Can you work these out from the model? Positions are in its coordinate system, mm. A direction names the side the tool comes from. Coordinates: 2 decimals unless noted, no trailing zeros. Order: outer loops, then holes, each group sorted by start corner. A loop starts at its lowest first (then second) coordinate and runs counter-clockwise, first axis right, second up. Notation, with made-up numbers: (32.5, 68) -> (51.5, 68) arc R6 cw to (51.5, 72) -> close; hole circle Ø11 at (-8, 37.5). An arc over 180 degrees is marked (long way). Write item = value, one per line. Start each with the question number.
Autodesk Inventor part; units mm, degrees
ref_plane "YZ Plane" through (0, 0, 0) normal (1, 0, 0) x (0, 1, 0)
ref_plane "XZ Plane" through (0, 0, 0) normal (0, 1, 0) x (-1, 0, 0)
ref_plane "XY Plane" through (0, 0, 0) normal (0, 0, 1) x (1, 0, 0)
sketch "Sketch1" plane through (0, 0, 0) normal (0, 1, 0) x (-1, 0, 0)
  line L0 (2, 0) -> (23, 0)
  line L1 (25, -2) -> (25, -21.862)
  line L2 (23, -23.862) -> (2, -23.862)
  line L3 (0, -21.862) -> (0, -2)
  arc A0 (25, -2) -> (23, 0) centre (23, -2) ccw
  arc A1 (23, -23.862) -> (25, -21.862) centre (23, -21.862) ccw
  arc A2 (0, -21.862) -> (2, -23.862) centre (2, -21.862) ccw
  arc A3 (2, 0) -> (0, -2) centre (2, -2) ccw
  line L4 (23, 0) -> (23, -23.862) construction
  line L5 (2, -23.862) -> (2, 0) construction
  line L6 (25, -2) -> (0, -2) construction
  line L7 (0, -14.5) -> (25, -14.5) construction
  circle A4 centre (23, -2) radius 1.1
  circle A5 centre (23, -14.5) radius 1.1
  circle A6 centre (2, -14.5) radius 1.1
  circle A7 centre (2, -2) radius 1.1
  point P0 (0, 0)
  point P1 (25, -23.862)
  point P2 (25, 0)
  point P3 (0, -23.862)
  dimension "d0" = 25
  dimension "d1" = 23.862
  dimension "d2" = 2
  dimension "d3" = 2
  dimension "d4" = 14.5
  dimension "d5" = 2
  dimension "d6" = 2
  dimension "d7" = 2.2
  dimension "d8" = 2.2
  dimension "d9" = 2.2
  dimension "d10" = 2.2
extrude "Extrusion1" add sketch "Sketch1" along normal blind 1.2
sketch "Sketch2" plane through (0, 1.2, 0) normal (0, 1, 0) x (1, 0, 0)
  line L0 (-25, 21.862) -> (-25, 2) construction
  line L1 (-25, 11.931) -> (0, 11.931) construction
  line L2 (0, 2) -> (0, 21.862) construction
  line L3 (-2, 23.862) -> (-23, 23.862) construction
  line L4 (-12.5, 23.862) -> (-12.5, 0) construction
  line L5 (-23, 0) -> (-2, 0) construction
  line L6 (-16.75, 18.65) -> (-8.25, 18.65)
  line L7 (-8.25, 18.65) -> (-8.25, 10.15)
  line L8 (-8.25, 10.15) -> (-16.75, 10.15)
  line L9 (-16.75, 10.15) -> (-16.75, 18.65)
  line L10 (-16.75, 14.4) -> (-8.25, 14.4) construction
  line L11 (-12.5, 18.65) -> (-12.5, 10.15) construction
  point P0 (0, 0)
  point P1 (-12.5, 14.4)
  dimension "d13" = 8.5
  dimension "d14" = 8.5
  dimension "d15" = 12.5
  dimension "d16" = 9.462
extrude "Extrusion2" add sketch "Sketch2" along normal blind 8
sketch "Sketch3" plane through (0, 0, 0) normal (0, -1, 0) x (1, 0, 0)
  line L0 (-2, -23.862) -> (-23, -23.862)
  line L1 (-22.9, -23.862) -> (-2.1, -23.862)
  line L2 (-2.1, -23.862) -> (-2.1, -18.362)
  line L3 (-2.1, -18.362) -> (-22.9, -18.362)
  line L4 (-22.9, -18.362) -> (-22.9, -23.862)
  line L5 (-12.5, -18.362) -> (-12.5, -23.862) construction
  point P0 (0, 0)
  dimension "d19" = 20.8
  dimension "d20" = 5.5
extrude "Extrusion3" add sketch "Sketch3" along normal blind 5
equation "\"d6\" = d5"
equation "\"d7\" = d8"
equation "\"d9\" = d8"
equation "\"d10\" = d8"
properties part number "RaspberryPiCamera"
(1) Imagine slicing it at D-D (x = -23.5). Write out the boundary of the cut face in (y, z).
(2) Thinking about a two-plate mould opening in Z: for faces 6 (the face through (-22.13, 0.59, -13.83)), 7 (the face through (-1.762, 0.592, -13.426)), 8 (the face through (-12, 1.2, -9)), 9 (the face through (-0.57, 0.59, -0.6)), which applies, +Z half, -Z half, draft (parallel to the pull), parting line (faces both ways), or undercut?
(3) Imagine slicing it at C-C (x = -7.75). Write out the boundary of the cut face in (y, z), plus the area to 3 significant figures.
(4) If I drill on L1, parallel to Z at x = -2, y = 0.5; L2, parallel to X at y = -1.25, z = -19.5; L3, parallel to Z at x = -8.75, y = -3, over which ranges is the centre line in solid material (lowest first)? Write a range as from..to.
(5) Imagine slicing it at A-A (z = -14.5). Write out the boundary of the cut face in (x, y), plus the area to 3 significant figures.
(6) For P1, Ø4, axis at y = 4.5, z = -16, coming from the -X side; P2, Ø2.5, axis at y = 6.5, z = -13.5, coming from the +X side; P3, Ø8, axis at x = -8, z = -10.5, coming from the -Y side; P4, Ø2, axis at x = -23, z = -2, coming from the -Y side, each with a flat end and sliding along its axis, tell me the tip position at first contact or that it passes through.
(7) For faces 1 (the face through (-12, -2, -18.362)), 2 (the face through (-22.9, -2, -21)), 3 (the face through (-13, 5, -18.65)), 4 (the face through (-12, 5, -10.15)), 5 (the face through (-2.1, -2, -21)), which set-ups out of +Z, -Z, +X, -X, +Y, -Y let a thin tool reach every point of the face, with its end or its side?
(8) Imagine slicing it at B-B (z = -10.5). Write out the boundary of the cut face in (x, y).
Result set:
q1.outline = (0, -23.8) -> (1.2, -23.8) -> (1.2, -15.48) -> (0, -15.48) -> close; (0, -13.52) -> (1.2, -13.52) -> (1.2, -2.98) -> (0, -2.98) -> close; (0, -1.02) -> (1.2, -1.02) -> (1.2, -0.06) -> (0, -0.06) -> close
q2.face_6 = undercut
q2.face_7 = undercut
q2.face_8 = draft
q2.face_9 = +Z half
q3.outline = (-5, -23.86) -> (1.2, -23.86) -> (1.2, 0) -> (0, 0) -> (0, -18.36) -> (-5, -18.36) -> close
q3.area = 56.1 mm2
q4.L1 = -23.86..-15.6, -13.4..-3.1, -0.9..0
q4.L2 = -22.9..-2.1
q4.L3 = -23.86..-18.36
q5.outline = (-25, 0) -> (-24.1, 0) -> (-24.1, 1.2) -> (-25, 1.2) -> close; (-21.9, 0) -> (-3.1, 0) -> (-3.1, 1.2) -> (-8.25, 1.2) -> (-8.25, 9.2) -> (-16.75, 9.2) -> (-16.75, 1.2) -> (-21.9, 1.2) -> close; (-0.9, 0) -> (0, 0) -> (0, 1.2) -> (-0.9, 1.2) -> close
q5.area = 92.7 mm2
q6.P1 = -16.75
q6.P2 = -8.25
q6.P3 = 0
q6.P4 = through
q7.face_1 = +Z, +X, -X, -Y
q7.face_2 = +Z, -Z, -X, -Y
q7.face_3 = -Z, +X, -X, +Y
q7.face_4 = +Z, +X, -X, +Y
q7.face_5 = +Z, -Z, +X, -Y
q8.outline = (-25, 0) -> (0, 0) -> (0, 1.2) -> (-8.25, 1.2) -> (-8.25, 9.2) -> (-16.75, 9.2) -> (-16.75, 1.2) -> (-25, 1.2) -> close
